Input: part model. Units: mm. Frame: model coordinates. A direction names the side the tool comes from. Coordinates: 2 decimals unless noted, no trailing zeros. Loops run counter-clockwise (first coordinate to the right, second up) from the corner with the lowest first, then second, coordinate; pieces in that order, holes last. Notation, with made-up numbers: M 43.25,-12.75 L 86.25,-12.75 A18 ccw 86.25,22.25 Z; hole C 43.25,-22.5 d2. An arc over 180 degrees is marked long. Use a Markdown table: item, result. Add a question column.
1. Pin query (flat end, axial travel): pin 1 (1 mm diameter, centred on x = 27, z = -5, fed in from -Y); pin 2 (3 mm diameter, centred on y = -1.5, z = -9.5, fed in from -X); pin 3 (1.5 mm diameter, centred on x = 18.5, y = 9.5, fed in from +Z); pin 4 (1.5 mm diameter, centred on x = 6, y = 7, fed in from -Z). Return the tip coordinate at first contact, or that it passes through.
2. Section B-B on y = -13. Output: boundary loops of the cut face in (x, z).
3. Section D-D on z = 13.5. Output: boundary loops of the cut face in (x, y).
4. Draft query along Z for faces 1 (the cylindrical face through (15.21, 16.627, -3.541)), 2 (the cylindrical face through (14.79, 12.83, 7.48)), 3 (the cylindrical face through (15.21, 1.783, 16.906)). Return one class per face: +Z half, -Z half, draft (parallel to the pull), parting line (faces both ways), or undercut.
5. Section A-A on z = 0. Output: boundary loops of the cut face in (x, y).
6. Line query: L1, parallel to Y at x = 9.5, z = 13; L2, parallel to Y at x = 14.5, z = 0; L3, parallel to Y at x = 3.5, z = -9. Output: solid intervals per line, ascending. Write a range as [from, to].
7. Set-up query: faces 4 (the cylindrical face through (14.79, -3.187, -14.572)), 5 (the cylindrical face through (14.79, -14.106, -4.651)), 6 (the cylindrical face through (14.8, 12.5, 0)), 7 (the cylindrical face through (14.79, 14.15, -4.53)). Return all of +Z, -Z, +X, -X, +Y, -Y with unobstructed straight access to the full face (end or side cutting, diameter ignored); none if empty.
8. Section C-C on y = 14.5. Output: boundary loops of the cut face in (x, z), then the cut area to 3 significant figures.
```python
from build123d import *

# Parameters (mm, degrees)
BASPROSKE_W              = 30
BASPROSKE_H              = 17
TOOTHCUT_DEPTH           = 39.444765573
TEETHCUTS_COUNT          = 15
TEETHCUTS_ANGLE          = 336
BORSKE_R                 = 5
BORE_DEPTH               = 50.0000508
ESBO_O1_R                = 5
RESSALTO_EXTRUS_O1_DEPTH = 30
CORTE_EXTRUS_O1_REACH    = 40.422


with BuildPart() as part:
    # BasProSke → Base-Revolve (revolve)
    with BuildSketch(Plane(origin=(0, 0, 0), x_dir=(1, 0, 0), z_dir=(0, 1, 0)), mode=Mode.PRIVATE) as base_revolve_sk:
        with Locations((15, 8.5)):
            Rectangle(BASPROSKE_W, BASPROSKE_H)
    revolve(base_revolve_sk.sketch.rotate(Axis((-10, 0, 0), (1, 0, 0)), 180), axis=Axis((-10, 0, 0), (1, 0, 0)))

    # TooCutSke → ToothCut (cut, through all)
    with BuildSketch(Plane(origin=(0, 0, 0), x_dir=(0, 0, -1), z_dir=(1, 0, 0))):
        with BuildLine():
            ThreePointArc((1.050056448, 12.454813626), (0, 12.499), (-1.050056448, 12.454813626))
            ThreePointArc((-1.050056448, 12.454813626), (-1.638118106, 14.809604533), (-3.110934279, 16.73876737))
            ThreePointArc((-3.110934279, 16.73876737), (0, 17.0254), (3.110934279, 16.73876737))
            ThreePointArc((3.110934279, 16.73876737), (1.638118106, 14.809604533), (1.050056448, 12.454813626))
        make_face()
    toothcut = extrude(amount=TOOTHCUT_DEPTH, mode=Mode.SUBTRACT)

    # TeethCuts: ToothCut ×15 about axis
    teethcuts_axis = Axis((-10, 0, 0), (1, 0, 0))
    for i in range(1, TEETHCUTS_COUNT):
        add(toothcut.rotate(teethcuts_axis, i * TEETHCUTS_ANGLE / (TEETHCUTS_COUNT - 1)), mode=Mode.SUBTRACT)

    # BorSke → Bore (cut, symmetric)
    with BuildSketch(Plane(origin=(0, 0, 0), x_dir=(0, 0, -1), z_dir=(1, 0, 0))):
        with Locations(Location((0, 0, 0), (0, 0, 180))):
            Circle(BORSKE_R)
    extrude(amount=BORE_DEPTH, both=True, mode=Mode.SUBTRACT)

    # Esboço1 → Ressalto-extrusão1 (add)
    with BuildSketch(Plane(origin=(30, 0, 0), x_dir=(0, 0, -1), z_dir=(1, 0, 0))):
        Circle(ESBO_O1_R)
    extrude(amount=-RESSALTO_EXTRUS_O1_DEPTH)

    # Esboço2 → Corte-extrusão1 (cut, up to next)
    with BuildSketch(Plane(origin=(30, 0, 0), x_dir=(0, 0, -1), z_dir=(1, 0, 0)), mode=Mode.PRIVATE) as corte_extrus_o1_sk1:
        with BuildLine():
            Line((-2.85, 1.341640786), (-2.85, -1.341640786))
            ThreePointArc((-2.85, -1.341640786), (3.15, 0), (-2.85, 1.341640786))
        make_face()
    corte_extrus_o1_tool1 = extrude(corte_extrus_o1_sk1.sketch, amount=-CORTE_EXTRUS_O1_REACH, mode=Mode.PRIVATE) & part.part
    add(corte_extrus_o1_tool1.solids().sort_by_distance((30, 0, -0.052561))[0], mode=Mode.SUBTRACT)


solid = part.part
```
Answers below:
| question | item | result |
|---|---|---|
| 1 | pin 1 | stops at y = -15.01 |
| 1 | pin 2 | stops at x = 0 |
| 1 | pin 3 | stops at z = 14.58 |
| 1 | pin 4 | stops at z = -14.78 |
| 2 | outline | M 0,-7.39 L 30,-7.39 L 30,-3.99 L 0,-3.99 Z; M 0,-1.63 L 30,-1.63 L 30,1.63 L 0,1.63 Z; M 0,3.99 L 30,3.99 L 30,7.39 L 0,7.39 Z |
| 3 | outline | M 0,-5.97 L 30,-5.97 L 30,-2.66 L 0,-2.66 Z; M 0,-0.24 L 30,-0.24 L 30,3.07 L 0,3.07 Z; M 0,6.06 L 30,6.06 L 30,8.93 L 0,8.93 Z |
| 4 | face 1 | -Z half |
| 4 | face 2 | undercut |
| 4 | face 3 | +Z half |
| 5 | outline | M 0,-17 L 30,-17 L 30,-3.15 L 0,-3.15 Z; M 0,3.15 L 30,3.15 L 30,12.5 L 0,12.5 Z |
| 6 | L1 | y = [-5.9, -2.5], [-0.27, 3.02], [5.65, 8.88] |
| 6 | L2 | y = [-17, -3.15], [3.15, 12.5] |
| 6 | L3 | y = [-10.32, 8.67], [9.6, 13.79] |
| 7 | face 4 | -Z, +X, -X |
| 7 | face 5 | +X, -X, -Y |
| 7 | face 6 | +X, -X, +Y |
| 7 | face 7 | +X, -X |
| 8 | outline | M 0,-4.51 L 30,-4.51 L 30,-1.5 L 0,-1.5 Z; M 0,1.5 L 30,1.5 L 30,4.51 L 0,4.51 Z |
| 8 | area | 181 mm² |
